from build123d import *

# Parameters (mm, degrees)
F0_R     = 27.7
F1_DEPTH = 20
F2_R     = 28.95
F3_DEPTH = 15


with BuildPart() as f1:
    # F0 (on Top) → F1 (new body)
    with BuildSketch(Plane.XY):
        with BuildLine():
            ThreePointArc((-7.087882, 34.951923), (-8.795551, 32.17859), (-11.517808, 30.390625))
            ThreePointArc((-11.517808, 30.390625), (-12.437212, 30.026085), (-13.345097, 29.633738))
            ThreePointArc((-13.345097, 29.633738), (-16.534306, 28.973093), (-19.702852, 29.726631))
            ThreePointArc((-19.702852, 29.726631), (-28.284271, 28.284271), (-29.726631, 19.702852))
            ThreePointArc((-29.726631, 19.702852), (-28.973093, 16.534306), (-29.633738, 13.345097))
            ThreePointArc((-29.633738, 13.345097), (-30.026085, 12.437212), (-30.390625, 11.517808))
            ThreePointArc((-30.390625, 11.517808), (-32.17859, 8.795551), (-34.951923, 7.087882))
            ThreePointArc((-34.951923, 7.087882), (-40, 0), (-34.951923, -7.087882))
            ThreePointArc((-34.951923, -7.087882), (-32.17859, -8.795551), (-30.390625, -11.517808))
            ThreePointArc((-30.390625, -11.517808), (-30.026085, -12.437212), (-29.633738, -13.345097))
            ThreePointArc((-29.633738, -13.345097), (-28.973093, -16.534306), (-29.726631, -19.702852))
            ThreePointArc((-29.726631, -19.702852), (-28.284271, -28.284271), (-19.702852, -29.726631))
            ThreePointArc((-19.702852, -29.726631), (-16.534306, -28.973093), (-13.345097, -29.633738))
            ThreePointArc((-13.345097, -29.633738), (-12.437212, -30.026085), (-11.517808, -30.390625))
            ThreePointArc((-11.517808, -30.390625), (-8.795551, -32.17859), (-7.087882, -34.951923))
            ThreePointArc((-7.087882, -34.951923), (0, -40), (7.087882, -34.951923))
            ThreePointArc((7.087882, -34.951923), (8.795551, -32.17859), (11.517808, -30.390625))
            ThreePointArc((11.517808, -30.390625), (12.437212, -30.026085), (13.345097, -29.633738))
            ThreePointArc((13.345097, -29.633738), (16.534306, -28.973093), (19.702852, -29.726631))
            ThreePointArc((19.702852, -29.726631), (28.284271, -28.284271), (29.726631, -19.702852))
            ThreePointArc((29.726631, -19.702852), (28.973093, -16.534306), (29.633738, -13.345097))
            ThreePointArc((29.633738, -13.345097), (30.026085, -12.437212), (30.390625, -11.517808))
            ThreePointArc((30.390625, -11.517808), (32.17859, -8.795551), (34.951923, -7.087882))
            ThreePointArc((34.951923, -7.087882), (40, 0), (34.951923, 7.087882))
            ThreePointArc((34.951923, 7.087882), (32.17859, 8.795551), (30.390625, 11.517808))
            ThreePointArc((30.390625, 11.517808), (30.026085, 12.437212), (29.633738, 13.345097))
            ThreePointArc((29.633738, 13.345097), (28.973093, 16.534306), (29.726631, 19.702852))
            ThreePointArc((29.726631, 19.702852), (28.284271, 28.284271), (19.702852, 29.726631))
            ThreePointArc((19.702852, 29.726631), (16.534306, 28.973093), (13.345097, 29.633738))
            ThreePointArc((13.345097, 29.633738), (12.437212, 30.026085), (11.517808, 30.390625))
            ThreePointArc((11.517808, 30.390625), (8.795551, 32.17859), (7.087882, 34.951923))
            ThreePointArc((7.087882, 34.951923), (0, 40), (-7.087882, 34.951923))
        make_face()
        Circle(F0_R, mode=Mode.SUBTRACT)
    extrude(amount=F1_DEPTH)

    # F2 (on face) → F3 (cut)
    with BuildSketch(Plane.XY.offset(20)):
        Circle(F2_R)
    extrude(amount=-F3_DEPTH, mode=Mode.SUBTRACT)


solid = f1.part
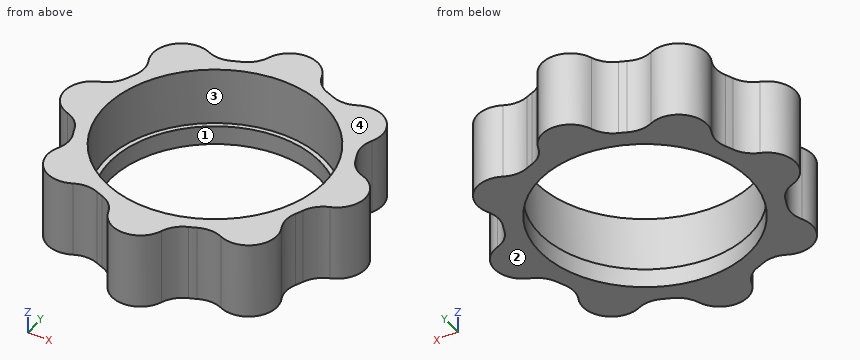
The model under review builds one solid part; all positions refer to its coordinate system, in mm. Face numbers are marked on the shaded views. A direction names the side the tool comes from. Coordinates: 2 decimals unless noted, no trailing zeros. Loops run counter-clockwise (first coordinate to the right, second up) from the corner with the lowest first, then second, coordinate; pieces in that order, holes last.
(1) Consider section D-D, the plane y = -31.5. Give the boundary of the cut face in (x, z).
Determined:
outline: (-9.55, 0) - (9.55, 0) - (9.55, 20) - (-9.55, 20) - close
(2) Wall thickness on L1, parallel to Y at x = 0, z = 15; L2, parallel to Y at x = 0, z = 2.85; L3, parallel to X at y = -25.5, z = 8.25: over which ranges is each line inside the solid? List them lowest first.
Determined:
L1: y = -40 to -28.95, 28.95 to 40
L2: y = -40 to -27.7, 27.7 to 40
L3: x = -30.05 to -13.71, 13.71 to 30.05
(3) Insertion check: P1, Ø1.5, axis at x = -17, z = 11, coming from the +Y side; P2, Ø1.5, axis at x = -24.5, z = 12.5, coming from the +Y side; P3, Ø8, axis at y = 18, z = 12, coming from the +X side. Each pin has a flat end and moves straight along its axis. Give the tip position at first contact, or say it passes through.
Determined:
P1: stops at y = 29.09
P2: stops at y = 30.44
P3: stops at x = 30.42
(4) Consider section A-A, the plane x = 0. Give the boundary of the cut face in (y, z).
Determined:
outline: (-40, 0) - (-27.7, 0) - (-27.7, 5) - (-28.95, 5) - (-28.95, 20) - (-40, 20) - close; (27.7, 0) - (40, 0) - (40, 20) - (28.95, 20) - (28.95, 5) - (27.7, 5) - close
(5) Draft analysis for pull direction X (two halves, no side actions). For the marked faces 1 and 2, state which applies: +X half, -X half, draft (parallel to the pull), parting line (faces both ways), or undercut.
Determined:
face 1: undercut
face 2: draft
(6) Tool access review of the marked faces 3 and 4: name each direction out of +Z, -Z, +X, -X, +Y, -Y from which nothing blocks a thin tool from reaching the whole face with its end or side.
Determined:
face 3: +Z
face 4: +Z, +X, -X, +Y, -Y
